```python
from build123d import *

# Parameters (mm, degrees)
BOSS_EXTRUDE1_DEPTH      = 4.5
BOSS_EXTRUDE1_DEPTH_BACK = 4.5
CUT_EXTRUDE1_DEPTH       = 2.7
CUT_EXTRUDE1_DEPTH_BACK  = 2.7
SKETCH2_R                = 8.25
SKETCH3_R                = 2
CUT_EXTRUDE3_DEPTH       = 24.484037132
CHAMFER1_SIZE            = 2


with BuildPart() as part:
    # Sketch1 → Boss-Extrude1 (new, two sides: drawn at the far end of the back side and taken through both)
    with BuildSketch(Plane(origin=(0, 0, 0), x_dir=(0, 0, -1), z_dir=(1, 0, 0)).offset(-BOSS_EXTRUDE1_DEPTH_BACK)):
        with BuildLine():
            Line((7, 7.5), (17.5, 7.5))
            Line((17.5, 7.5), (17.5, -7.5))
            Line((17.5, -7.5), (-17.5, -7.5))
            Line((-17.5, -7.5), (-17.5, 7.5))
            Line((-17.5, 7.5), (-7, 7.5))
            ThreePointArc((-7, 7.5), (0, 0.5), (7, 7.5))
        make_face()
    extrude(amount=BOSS_EXTRUDE1_DEPTH + BOSS_EXTRUDE1_DEPTH_BACK)

    # Sketch2 → Cut-Extrude1 (cut, two sides: drawn at the far end of the back side and taken through both)
    with BuildSketch(Plane(origin=(0, 0, 0), x_dir=(0, 0, -1), z_dir=(1, 0, 0)).offset(-CUT_EXTRUDE1_DEPTH_BACK)):
        with Locations((0, 7.5)):
            Circle(SKETCH2_R)
    extrude(amount=CUT_EXTRUDE1_DEPTH + CUT_EXTRUDE1_DEPTH_BACK, mode=Mode.SUBTRACT)

    # Sketch3 → Cut-Extrude3 (cut, through all)
    with BuildSketch(Plane(origin=(0, 7.5, 0), x_dir=(1, 0, 0), z_dir=(0, 1, 0))):
        with Locations(Location((0, 12.5, 0), (0, 0, 270))):
            Circle(SKETCH3_R)
        with Locations(Location((0, -12.5, 0), (0, 0, 270))):
            Circle(SKETCH3_R)
    extrude(amount=-CUT_EXTRUDE3_DEPTH, mode=Mode.SUBTRACT)

    # Chamfer1
    chamfer1_edges = [part.edges().sort_by_distance(p)[0] for p in [
        (0, 7.5, 17.5),
        (0, 7.5, -17.5),
    ]]
    chamfer(chamfer1_edges, length=CHAMFER1_SIZE)


solid = part.part
```
Verification items for the finished model (mm, model axes). A direction names the side the tool comes from. Round coordinates to 2 decimals unless told otherwise and drop trailing zeros. Write each loop counter-clockwise with the first axis right and the second up, starting at its lowest first coordinate (ties: lowest second). Pieces come first, ordered by that corner, then holes.
1. Section check D-D on z = 0. Enter the section's corners in (x, y).
2. Draft check along Z on faces 3 (the cylindrical face through (-1.2, 0.1, 10.9)), 4 (the flat face through (0, -1, -17.5)), 5 (the flat face through (0, 7.5, -10)). Enter one of: +Z half, -Z half, draft (parallel to the pull), parting line (faces both ways), or undercut.
3. Section check A-A on z = -12.5. Enter the section's corners in (x, y).
4. Section check B-B on y = 2.5. Enter the section's corners in (x, z).
5. Scan lines: L1, parallel to X at y = -0.25, z = 12.5; L2, parallel to Z at x = -1.5, y = 6; L3, parallel to Z at x = 1, y = -3.5. Record each from-to range of solid material in increasing order.
6. Section check C-C on x = -0.5. Enter the section's corners in (y, z), plus the area to 3 significant figures.
7. Access from +Z, -Z, +X, -X, +Y, -Y to the whole of each face (thin tool, end or side, straight path). Record for faces 1 (the flat face through (-4.5, 0, 0)), 2 (the flat face through (-2.7, 0, 0)).
8. Gauge pin test, flat end, axial feed: P1, Ø4.5, axis at x = 0, z = -12.5, coming from the -Y side. Record the tip position at first contact, or that the pin passes through.
Answer:
1. outline: (-4.5, -7.5) - (4.5, -7.5) - (4.5, 0.5) - (2.7, 0.5) - (2.7, -0.75) - (-2.7, -0.75) - (-2.7, 0.5) - (-4.5, 0.5) - close
2. face 3: undercut
2. face 4: -Z half
2. face 5: draft
3. outline: (-4.5, -7.5) - (-2, -7.5) - (-2, 7.5) - (-4.5, 7.5) - close; (2, -7.5) - (4.5, -7.5) - (4.5, 7.5) - (2, 7.5) - close
4. outline: (-4.5, -17.5) - (4.5, -17.5) - (4.5, -4.9) - (2.7, -4.9) - (2.7, -6.56) - (-2.7, -6.56) - (-2.7, -4.9) - (-4.5, -4.9) - close; (-4.5, 4.9) - (-2.7, 4.9) - (-2.7, 6.56) - (2.7, 6.56) - (2.7, 4.9) - (4.5, 4.9) - (4.5, 17.5) - (-4.5, 17.5) - close; hole circle Ø4 at (0, -12.5); hole circle Ø4 at (0, 12.5)
5. L1: x = -4.5 to -2, 2 to 4.5
5. L2: z = -17 to -13.82, -11.18 to -8.11, 8.11 to 11.18, 13.82 to 17
5. L3: z = -17.5 to -14.23, -10.77 to 10.77, 14.23 to 17.5
6. outline: (-7.5, -17.5) - (5.5, -17.5) - (7.5, -15.5) - (7.5, -14.44) - (-7.5, -14.44) - close; (-7.5, -10.56) - (7.5, -10.56) - (7.5, -8.25) arc R8.25 cw to (7.5, 8.25) - (7.5, 10.56) - (-7.5, 10.56) - close; (-7.5, 14.44) - (7.5, 14.44) - (7.5, 15.5) - (5.5, 17.5) - (-7.5, 17.5) - close
6. area: 298 mm2
7. face 1: +Z, -Z, -X, +Y, -Y
7. face 2: +Y
8. P1: stops at y = -7.5
